```python
from build123d import *

# Parameters (mm, degrees)
SKETCH1_W            = 40
SKETCH1_H            = 48.8
BOSS_EXTRUDE1_DEPTH  = 5
SKETCH2_W            = 20.5
SKETCH2_H            = 8
CUT_EXTRUDE1_DEPTH   = 6
SKETCH3_R            = 2.7
CUT_EXTRUDE2_DEPTH   = 2.8
SKETCH5_R            = 1
CUT_EXTRUDE3_DEPTH   = 6
SKETCH6_OUTSIDE_W    = 63.46
SKETCH6_OUTSIDE_H    = 19.66
CUT_EXTRUDE4_DEPTH   = 41
SKETCH7_OUTSIDE_W    = 54.66
SKETCH7_OUTSIDE_H    = 19.66
CUT_EXTRUDE5_DEPTH   = 49.8
SKETCH8_W            = 17.65
SKETCH8_H            = 28.05
CUT_EXTRUDE6_DEPTH   = 6
BOSS_EXTRUDE2_REACH  = 7
SKETCH9_W            = 2.93050761
SKETCH9_H            = 5
SKETCH9_W_2          = 3
SKETCH10_W           = 35.8
SKETCH10_H           = 38
CUT_EXTRUDE7_DEPTH   = 0.8
SKETCH11_W           = 36
SKETCH11_H           = 24
CUT_EXTRUDE8_DEPTH   = 2.8
SKETCH12_W           = 4
SKETCH12_H           = 26.7
CUT_EXTRUDE9_DEPTH   = 3.3
SKETCH13_OUTSIDE_W   = 54.66
SKETCH13_OUTSIDE_H   = 63.46
SKETCH13_OUTSIDE_W_2 = 40
SKETCH13_OUTSIDE_H_2 = 48.8
CUT_EXTRUDE10_DEPTH  = 3.3
SKETCH14_W           = 3.8
SKETCH14_H           = 4.5
FILLET1_R            = 2


with BuildPart() as part:
    # Sketch1 → Boss-Extrude1 (new body)
    with BuildSketch(Plane(origin=(0, 0, 0), x_dir=(1, 0, 0), z_dir=(0, 1, 0))):
        with Locations((-15.144927536, 0.78115942)):
            Rectangle(SKETCH1_W, SKETCH1_H)
    extrude(amount=BOSS_EXTRUDE1_DEPTH)

    # Sketch2 → Cut-Extrude1 (cut, through all)
    with BuildSketch(Plane(origin=(0, 5, 0), x_dir=(1, 0, 0), z_dir=(0, 1, 0))):
        with Locations((-15.144927536, -23.61884058)):
            Rectangle(SKETCH2_W, SKETCH2_H)
        with Locations((-15.144927536, 25.18115942)):
            Rectangle(SKETCH2_W, SKETCH2_H)
    extrude(amount=-CUT_EXTRUDE1_DEPTH, mode=Mode.SUBTRACT)

    # Sketch3 → Cut-Extrude2 (cut)
    with BuildSketch(Plane(origin=(0, 5, 0), x_dir=(1, 0, 0), z_dir=(0, 1, 0))):
        with Locations((-30.144927536, 16.18115942)):
            Circle(SKETCH3_R)
        with Locations((-0.144927536, 16.18115942)):
            Circle(SKETCH3_R)
        with Locations((-30.144927536, -14.61884058)):
            Circle(SKETCH3_R)
        with Locations((-0.144927536, -14.61884058)):
            Circle(SKETCH3_R)
    extrude(amount=-CUT_EXTRUDE2_DEPTH, mode=Mode.SUBTRACT)

    # Sketch5 → Cut-Extrude3 (cut, through all)
    with BuildSketch(Plane(origin=(0, 5, 0), x_dir=(1, 0, 0), z_dir=(0, 1, 0))):
        with Locations((-30.144927536, -14.61884058)):
            Circle(SKETCH5_R)
        with Locations((-0.144927536, -14.61884058)):
            Circle(SKETCH5_R)
        with Locations((-0.144927536, 16.18115942)):
            Circle(SKETCH5_R)
        with Locations((-30.144927536, 16.18115942)):
            Circle(SKETCH5_R)
    extrude(amount=-CUT_EXTRUDE3_DEPTH, mode=Mode.SUBTRACT)

    # Sketch6 outside → Cut-Extrude4 (cut, through all)
    with BuildSketch(Plane(origin=(4.855072464, 0, 0), x_dir=(0, 0, -1), z_dir=(1, 0, 0))):
        with Locations((0.781, 2.5)):
            Rectangle(SKETCH6_OUTSIDE_W, SKETCH6_OUTSIDE_H)
        Polygon((-18.61884058, 5), (-23.61884058, 1.5), (-23.61884058, 0), (25.18115942, 0), (25.18115942, 1.5), (20.18115942, 5), align=None, mode=Mode.SUBTRACT)
    extrude(amount=-CUT_EXTRUDE4_DEPTH, mode=Mode.SUBTRACT)

    # Sketch7 outside → Cut-Extrude5 (cut, through all)
    with BuildSketch(Plane.XY.offset(23.61884058)):
        with Locations((-15.145, 2.5)):
            Rectangle(SKETCH7_OUTSIDE_W, SKETCH7_OUTSIDE_H)
        Polygon((4.855072464, 1.5), (3.355072464, 5), (-33.644927536, 5), (-35.144927536, 1.5), (-35.144927536, 0), (4.855072464, 0), align=None, mode=Mode.SUBTRACT)
    extrude(amount=-CUT_EXTRUDE5_DEPTH, mode=Mode.SUBTRACT)

    # Sketch8 → Cut-Extrude6 (cut, through all)
    with BuildSketch(Plane(origin=(0, 5, 0), x_dir=(1, 0, 0), z_dir=(0, 1, 0))):
        with Locations((-15.119927536, 0.80615942)):
            Rectangle(SKETCH8_W, SKETCH8_H)
    extrude(amount=-CUT_EXTRUDE6_DEPTH, mode=Mode.SUBTRACT)

    # Sketch9 → Boss-Extrude2 (add, up to next)
    with BuildSketch(Plane(origin=(0, 5, 0), x_dir=(1, 0, 0), z_dir=(0, 1, 0)), mode=Mode.PRIVATE) as boss_extrude2_sk1:
        with Locations((3.355072464, 10.36115942)):
            Rectangle(SKETCH9_W, SKETCH9_H)
    boss_extrude2_tool1 = extrude(boss_extrude2_sk1.sketch, amount=-BOSS_EXTRUDE2_REACH, mode=Mode.PRIVATE) - part.part
    add(boss_extrude2_tool1.solids().sort_by_distance((3.355072, 5, -10.361159))[0])
    # Sketch9 → Boss-Extrude2 (add, up to next)
    with BuildSketch(Plane(origin=(0, 5, 0), x_dir=(1, 0, 0), z_dir=(0, 1, 0)), mode=Mode.PRIVATE) as boss_extrude2_sk2:
        with Locations((3.355072464, 3.96115942)):
            Rectangle(SKETCH9_W, SKETCH9_H)
    boss_extrude2_tool2 = extrude(boss_extrude2_sk2.sketch, amount=-BOSS_EXTRUDE2_REACH, mode=Mode.PRIVATE) - part.part
    add(boss_extrude2_tool2.solids().sort_by_distance((3.355072, 5, -3.961159))[0])
    # Sketch9 → Boss-Extrude2 (add, up to next)
    with BuildSketch(Plane(origin=(0, 5, 0), x_dir=(1, 0, 0), z_dir=(0, 1, 0)), mode=Mode.PRIVATE) as boss_extrude2_sk3:
        with Locations((3.355072464, -2.33884058)):
            Rectangle(SKETCH9_W, SKETCH9_H)
    boss_extrude2_tool3 = extrude(boss_extrude2_sk3.sketch, amount=-BOSS_EXTRUDE2_REACH, mode=Mode.PRIVATE) - part.part
    add(boss_extrude2_tool3.solids().sort_by_distance((3.355072, 5, 2.338841))[0])
    # Sketch9 → Boss-Extrude2 (add, up to next)
    with BuildSketch(Plane(origin=(0, 5, 0), x_dir=(1, 0, 0), z_dir=(0, 1, 0)), mode=Mode.PRIVATE) as boss_extrude2_sk4:
        with Locations((3.355072464, -8.61884058)):
            Rectangle(SKETCH9_W, SKETCH9_H)
    boss_extrude2_tool4 = extrude(boss_extrude2_sk4.sketch, amount=-BOSS_EXTRUDE2_REACH, mode=Mode.PRIVATE) - part.part
    add(boss_extrude2_tool4.solids().sort_by_distance((3.355072, 5, 8.618841))[0])
    # Sketch9 → Boss-Extrude2 (add, up to next)
    with BuildSketch(Plane(origin=(0, 5, 0), x_dir=(1, 0, 0), z_dir=(0, 1, 0)), mode=Mode.PRIVATE) as boss_extrude2_sk5:
        with Locations((-33.644927536, -8.61884058)):
            Rectangle(SKETCH9_W_2, SKETCH9_H)
    boss_extrude2_tool5 = extrude(boss_extrude2_sk5.sketch, amount=-BOSS_EXTRUDE2_REACH, mode=Mode.PRIVATE) - part.part
    add(boss_extrude2_tool5.solids().sort_by_distance((-33.644928, 5, 8.618841))[0])

    # Sketch10 → Cut-Extrude7 (cut)
    with BuildSketch(Plane.XZ):
        with Locations((-15.144927536, -0.78115942)):
            Rectangle(SKETCH10_W, SKETCH10_H)
    extrude(amount=-CUT_EXTRUDE7_DEPTH, mode=Mode.SUBTRACT)

    # Sketch11 → Cut-Extrude8 (cut)
    with BuildSketch(Plane.XZ):
        with Locations((-15.144927536, -0.78115942)):
            Rectangle(SKETCH11_W, SKETCH11_H)
    extrude(amount=-CUT_EXTRUDE8_DEPTH, mode=Mode.SUBTRACT)

    # Sketch12 → Cut-Extrude9 (cut)
    with BuildSketch(Plane.XZ):
        with Locations((-5.144927536, -0.93115942)):
            Rectangle(SKETCH12_W, SKETCH12_H)
    extrude(amount=-CUT_EXTRUDE9_DEPTH, mode=Mode.SUBTRACT)

    # Sketch13 outside → Cut-Extrude10 (cut)
    with BuildSketch(Plane.XZ):
        with Locations((-15.145, -0.781)):
            Rectangle(SKETCH13_OUTSIDE_W, SKETCH13_OUTSIDE_H)
        with Locations((-15.144927536, -0.78115942)):
            Rectangle(SKETCH13_OUTSIDE_W_2, SKETCH13_OUTSIDE_H_2, mode=Mode.SUBTRACT)
        Polygon((2.855072464, -13.18115942), (-3.144927536, -13.18115942), (-3.144927536, -19.776149343), (-27.144927536, -19.78115942), (-27.144927536, -13.18115942), (-33.144927536, -13.18115942), (-33.144927536, 11.61884058), (-27.144927536, 11.61884058), (-27.144927536, 18.21884058), (-3.144927536, 18.21884058), (-3.144927536, 11.61884058), (2.855072464, 11.61884058), align=None)
    extrude(amount=-CUT_EXTRUDE10_DEPTH, mode=Mode.SUBTRACT)

    # Sketch14 → Cut-Revolve1 (revolve, cut)
    with BuildSketch(Plane.XZ):
        with Locations((-32.544927536, -10.73115942)):
            Rectangle(SKETCH14_W, SKETCH14_H)
    revolve(axis=Axis((-30.644927536, 0, -16.414338521), (0, 0, 1)), mode=Mode.SUBTRACT)

    # Fillet1
    fillet1_edges = [part.edges().sort_by_distance(p)[0] for p in [
        (-3.144927536, 2.05, -13.18115942),
        (-27.144927536, 2.05, -13.18115942),
        (-27.144927536, 2.05, 11.61884058),
        (-3.144927536, 2.05, 11.61884058),
    ]]
    fillet(fillet1_edges, radius=FILLET1_R)


solid = part.part
```
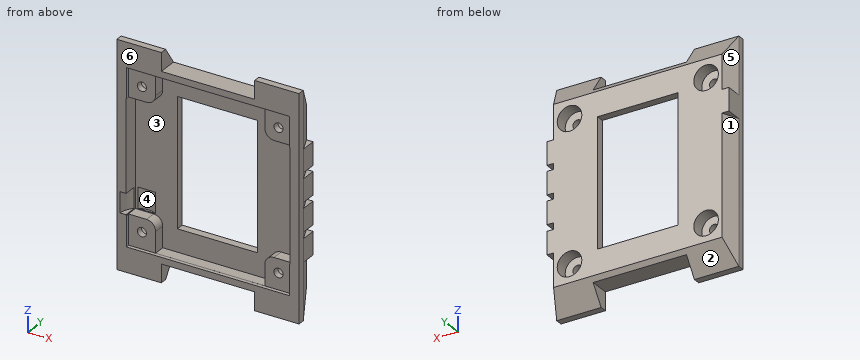
Source: CAD feature listing. Evaluate the final solid. Frame: model axes, mm. Face numbers are marked on the shaded views. A direction names the side the tool comes from. Coordinates: 2 decimals unless noted, no trailing zeros. Loops run counter-clockwise (first coordinate to the right, second up) from the corner with the lowest first, then second, coordinate; pieces in that order, holes last. Notation, with made-up numbers: M 56,-3.75 L 82,-3.75 A22 cw 82,7.25 Z; hole C -16,45.5 d7. An arc over 180 degrees is marked long. Use a Markdown table: item, result. Add a question column.
Q1. Section query A-A, the plane z = -9.5. Return loops of the section in (x, y).
Q2. Access query for the marked faces 4, 5 and 6. Directions: +Z, -Z, +X, -X, +Y, -Y. A direction counts if a zero-diameter tool reaches every point of the face in a straight line with its end or side. Return the directions, or none.
Q3. First-contact query: pin 1 (3 mm diameter, centred on x = -20.5, y = 2, fed in from +Z); pin 2 (3 mm diameter, centred on x = -26, z = -2, fed in from -Y); pin 3 (5 mm diameter, centred on x = -30.14, z = 14.62, fed in from +Y). Flat tips, straight axial feed; report the tip coordinate or a pass-through.
Q4. Draft query along X for the marked faces 1, 2 and 3. Return one class per face: pulls with the +X half, pulls with the -X half, needs draft (parallel to the pull), parting line crosses it, or undercut.
Q5. Section query D-D, the plane z = 12.5. Return loops of the section in (x, y).
Q6. Material intervals for L1, parallel to Z at x = -21, y = 3.9; L2, parallel to Z at x = -10, y = 3.25; L3, parallel to X at y = 2.1, z = -16, sorted ascending.
Result:
| question | item | result |
|---|---|---|
| 1 | outline | M -35.14,0 L -34.44,0 A3.8 cw -33.14,2.86 L -33.14,3.3 L -32.53,3.3 A3.8 cw -28.76,3.3 L -23.94,3.3 L -23.94,5 L -33.64,5 L -35.14,1.5 Z; M -6.29,3.3 L 2.86,3.3 L 2.86,0 L 4.86,0 L 4.86,1.5 L 4.82,1.58 L 4.82,5 L -6.29,5 Z |
| 2 | face 4 | -Y |
| 2 | face 5 | +Z, -X, +Y |
| 2 | face 6 | +Z, -Z, +X, -X, -Y |
| 3 | pin 1 | stops at z = 19.62 |
| 3 | pin 2 | stops at y = 3.3 |
| 3 | pin 3 | stops at y = 2.2 |
| 4 | face 1 | pulls with the -X half |
| 4 | face 2 | needs draft |
| 4 | face 3 | undercut |
| 5 | outline | M -35.14,0 L -33.04,0 L -33.04,0.8 L -27.49,0.8 L -27.49,3.3 L -23.94,3.3 L -23.94,5 L -28.47,5 L -28.47,2.2 L -31.82,2.2 L -31.82,5 L -33.64,5 L -35.14,1.5 Z; M -6.29,3.3 L -2.8,3.3 L -2.8,0.8 L 2.76,0.8 L 2.76,0 L 4.86,0 L 4.86,1.5 L 3.36,5 L 1.53,5 L 1.53,2.2 L -1.82,2.2 L -1.82,5 L -6.29,5 Z |
| 6 | L1 | z = -21.18 to -14.83, 13.22 to 19.62 |
| 6 | L2 | z = -21.18 to -19.78, 18.22 to 19.62 |
| 6 | L3 | x = -34.89 to -31.13, -29.16 to -27.14, -3.14 to -1.13, 0.84 to 4.6 |
